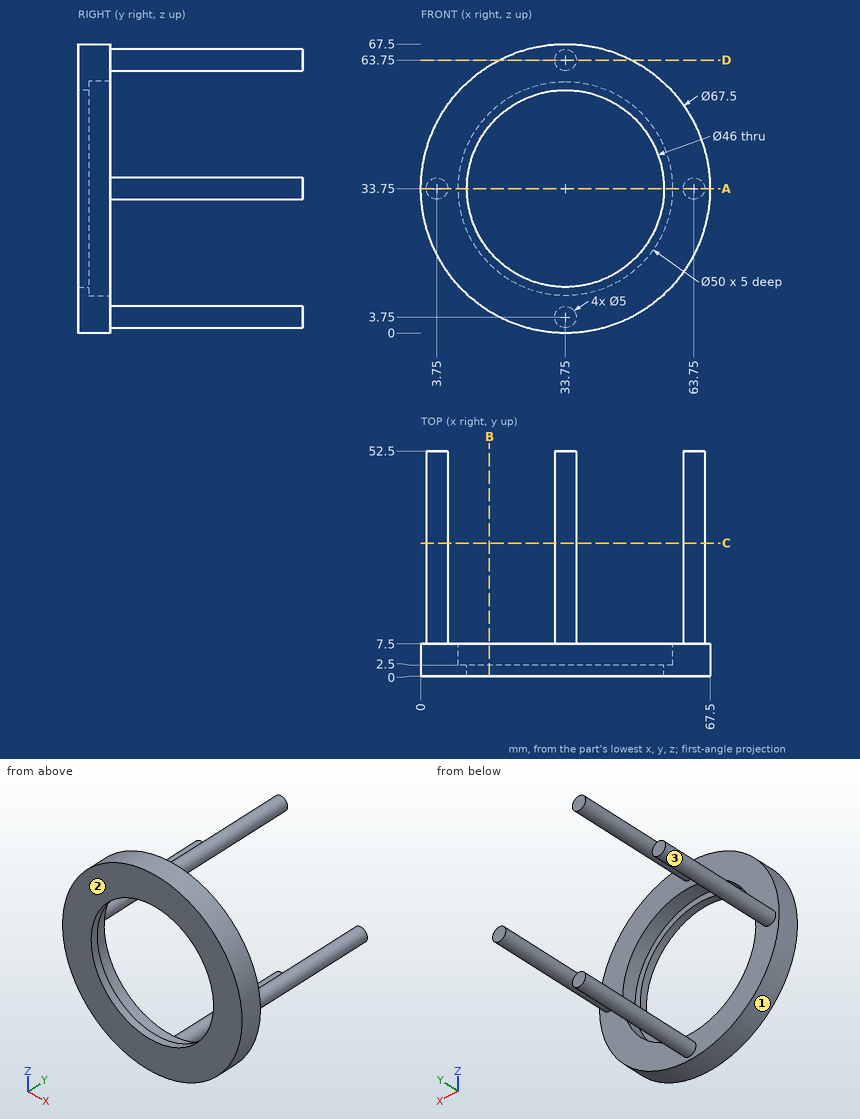
Part print with two shaded views. Sizes in mm from the minimum x, y, z corner. Round coordinates to 2 decimals unless told otherwise and drop trailing zeros. Order: outer loops, then holes, each group sorted by start corner. A loop starts at its lowest first (then second) coordinate and runs counter-clockwise, first axis right, second up. Notation, with made-up numbers: (72, -7.75) - (114, -7.75) arc R30 cw to (114, 17.25) - close; hole circle Ø5 at (-13.75, 15.25). An arc over 180 degrees is marked (long way). Answer in a Markdown table with one row per item. Add a question column.
(1) Drop flat-ended pins along their axis: pin 1 Ø12 at (y, z) = (7, 33) entering from +X; pin 2 Ø3 at (x, z) = (18.5, 54.5) entering from +Y; pin 3 Ø10 at (y, z) = (30, 40.5) entering from -X. Give the stop position or say it passes through.
(2) Band-saw the part on C-C on y = 31. List the corners of the cut face in (x, z), and give its area (3 significant figures).
(3) Mould opens along X. For the marked faces 1, 2 and 3 say: +X half, -X half, draft (parallel to the pull), parting line (faces both ways), or undercut.
(4) Band-saw the part on A-A on z = 33.75. List the corners of the cut face in (x, y), and give its area (3 significant figures).
(5) Band-saw the part on D-D on z = 63.75. List the corners of the cut face in (x, y).
(6) Band-saw the part on B-B on x = 16. List the corners of the cut face in (y, z).
(7) Probe L1, parallel to X at y = 1, z = 33.75; L2, parallel to X at y = 49.5, z = 34; L3, parallel to Z at x = 33, y = 6. List the from-to ranges inside material, lowest first. Write a range as [from, to].
Data:
| question | item | result |
|---|---|---|
| 1 | pin 1 | stops at x = 67.5 |
| 1 | pin 2 | stops at y = 7.5 |
| 1 | pin 3 | stops at x = 1.96 |
| 2 | outline | circle Ø5 at (3.75, 33.75); circle Ø5 at (33.75, 3.75); circle Ø5 at (33.75, 63.75); circle Ø5 at (63.75, 33.75) |
| 2 | area | 78.5 mm^2 |
| 3 | face 1 | parting line |
| 3 | face 2 | draft |
| 3 | face 3 | undercut |
| 4 | outline | (0, 0) - (10.75, 0) - (10.75, 2.5) - (8.75, 2.5) - (8.75, 7.5) - (6.25, 7.5) - (6.25, 52.5) - (1.25, 52.5) - (1.25, 7.5) - (0, 7.5) - close; (56.75, 0) - (67.5, 0) - (67.5, 7.5) - (66.25, 7.5) - (66.25, 52.5) - (61.25, 52.5) - (61.25, 7.5) - (58.75, 7.5) - (58.75, 2.5) - (56.75, 2.5) - close |
| 4 | area | 591 mm^2 |
| 5 | outline | (18.29, 0) - (49.21, 0) - (49.21, 7.5) - (36.25, 7.5) - (36.25, 52.5) - (31.25, 52.5) - (31.25, 7.5) - (18.29, 7.5) - close |
| 6 | outline | (0, 5.04) - (7.5, 5.04) - (7.5, 16.14) - (2.5, 16.14) - (2.5, 19.12) - (0, 19.12) - close; (0, 48.38) - (2.5, 48.38) - (2.5, 51.36) - (7.5, 51.36) - (7.5, 62.46) - (0, 62.46) - close |
| 7 | L1 | x = [0, 10.75], [56.75, 67.5] |
| 7 | L2 | x = [1.26, 6.24], [61.26, 66.24] |
| 7 | L3 | z = [0.01, 8.76], [58.74, 67.49] |
